Could you check a few things on this model? Use its own coordinates, in mm. Face numbers are marked on the shaded views. A direction names the side the tool comes from. Coordinates: 2 decimals unless noted, no trailing zeros. Order: outer loops, then holes, each group sorted by start corner. A loop starts at its lowest first (then second) coordinate and runs counter-clockwise, first axis right, second up. Notation, with made-up numbers: M 36,28.5 L 62,28.5 A20 ccw 62,38.5 Z; hole C 65.25,-3 d10. An arc over 180 degrees is marked long. One line per question, with ' | ' between items. Start each with the question number.
from build123d import *

# Parameters (mm, degrees)
EXTRUDE_1_DEPTH     = 11.5
FILLET_1_R          = 1
EXTRUDE_2_DEPTH     = 3.2
CUT_EXTRUDE_1_DEPTH = 1.8
CUT_EXTRUDE_2_DEPTH = 1.4


with BuildPart() as part:
    # 草图1 → 凸台-拉伸1 (new body)
    with BuildSketch(Plane(origin=(0, 0, 0), x_dir=(0, 0, -1), z_dir=(1, 0, 0))):
        Polygon((5.9, 0), (5.9, 9.85), (-5.9, 9.85), (-5.9, 0), (-7.2, 0), (-7.2, 11.15), (7.2, 11.15), (7.2, 0), align=None)
    extrude(amount=EXTRUDE_1_DEPTH)

    # 圆角1
    fillet_1_edges = [part.edges().sort_by_distance(p)[0] for p in [
        (5.75, 11.15, 7.2),
        (5.75, 11.15, -7.2),
        (5.75, 9.85, -5.9),
        (5.75, 9.85, 5.9),
    ]]
    fillet(fillet_1_edges, radius=FILLET_1_R)

    # 草图2 → 凸台-拉伸2 (add)
    with BuildSketch(Plane(origin=(0, 0, 0), x_dir=(1, 0, 0), z_dir=(0, 1, 0))):
        with BuildLine():
            Line((0, -7.2), (0, -8.8))
            ThreePointArc((0, -8.8), (4.2, -13), (8.4, -8.8))
            Line((8.4, -8.8), (8.4, -7.2))
            Line((8.4, -7.2), (0, -7.2))
        make_face()
    extrude_2 = extrude(amount=EXTRUDE_2_DEPTH)

    # 草图10 → 切除-拉伸1 (cut)
    with BuildSketch(Plane(origin=(0, 3.2, 0), x_dir=(1, 0, 0), z_dir=(0, 1, 0))):
        Polygon((7.085479679, -8.8), (6.161719249, -7.2), (2.235737418, -7.2), (1.311976987, -8.8), (2.75535266, -11.3), (5.642104006, -11.3), align=None)
    cut_extrude_1 = extrude(amount=-CUT_EXTRUDE_1_DEPTH, mode=Mode.SUBTRACT)

    # 草图11 → 切除-拉伸2 (cut)
    with BuildSketch(Plane(origin=(0, 0, 0), x_dir=(1, 0, 0), z_dir=(0, 1, 0))):
        with BuildLine():
            Line((3.087032009, -8.8), (3.087032009, -4.948738573))
            Line((3.087032009, -4.948738573), (5.337032009, -4.948738573))
            Line((5.337032009, -4.948738573), (5.337032009, -8.8))
            ThreePointArc((5.337032009, -8.8), (4.212032009, -9.925), (3.087032009, -8.8))
        make_face()
    cut_extrude_2 = extrude(amount=CUT_EXTRUDE_2_DEPTH, mode=Mode.SUBTRACT)

    # 镜向1: 凸台-拉伸2, 切除-拉伸1, 切除-拉伸2 across plane
    add(extrude_2.mirror(Plane.XY))
    add(cut_extrude_1.mirror(Plane.XY), mode=Mode.SUBTRACT)
    add(cut_extrude_2.mirror(Plane.XY), mode=Mode.SUBTRACT)


solid = part.part
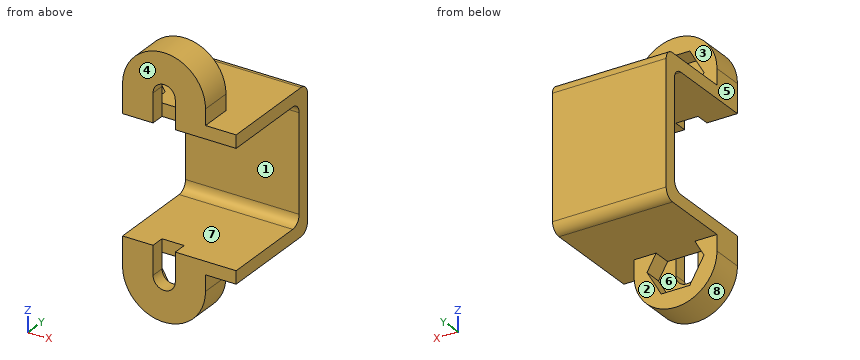
(1) Imagine slicing it at D-D, the plane z = -7.75. Write out the boundary of the cut face in (x, y), plus the area to 3 significant figures.
(2) Imagine slicing it at C-C, the plane x = 8.75. Write out the boundary of the cut face in (y, z).
(3) On a 3-axis mill with a long thin cutter (end or side, diameter ignored), from which of +Z, -Z, +X, -X, +Y, -Y can I reach the whole of each face in a straight line? I mean the marked faces 1, 2, 3 and 4. Say none if no direction works.
(4) For P1, Ø6, axis at x = 9.5, z = 3, coming from the -Y side; P2, Ø4.5, axis at x = 6, y = 6, coming from the +Z side; P3, Ø1.2, axis at x = 5, z = 8.5, coming from the +Y side; P4, Ø5, axis at x = 3.5, z = 2.5, coming from the -Y side (3 decimals), each with a flat end and sliding along its axis, tell me the tip position at first contact or that it passes through.
(5) If I drill on line 1 along Z through (x, y) = (6, 7); line 2 along Y through (x, z) = (9.25, -3.25); line 3 along X through (y, z) = (1.25, -6), over which ranges is the centre line in solid material (lowest first)? Write a range as from..to.
(6) Imagine slicing it at A-A, the plane y = 1.75. Write out the boundary of the cut face in (x, z), plus the area to 3 significant figures.
(7) We'd pull the mould along X, two halves only. Please class the marked faces 5, 6, 7 and 8: +X half, -X half, draft (parallel to the pull), parting line (faces both ways), or undercut.
(8) Imagine slicing it at B-B, the plane x = 4.2. Write out the boundary of the cut face in (y, z), plus the area to 3 significant figures.
Answers:
1) outline: M 0,0 L 3.09,0 L 3.09,1.4 L 1.92,1.4 L 1.92,3.2 L 0,3.2 Z; M 5.34,0 L 8.4,0 L 8.4,3.2 L 6.48,3.2 L 6.48,1.4 L 5.34,1.4 Z | area: 15.5 mm²
2) outline: M 0,-7.2 L 10.15,-7.2 A1 ccw 11.15,-6.2 L 11.15,6.2 A1 ccw 10.15,7.2 L 0,7.2 L 0,5.9 L 8.85,5.9 A1 cw 9.85,4.9 L 9.85,-4.9 A1 cw 8.85,-5.9 L 0,-5.9 Z
3) face 1: +X, -X, -Y | face 2: -Z, +X, -X, +Y | face 3: +Z, +X, -X, +Y | face 4: +Z, -Z, +X, -X, -Y
4) P1: y = 0 | P2: z = 7.2 | P3: y = 1.4 | P4: y = 9.845
5) line 1: -7.2..-5.9, 5.9..7.2 | line 2: 9.85..11.15 | line 3: 0..3.09, 5.34..11.5
6) outline: M 0,-8.8 A4.2 ccw 8.4,-8.8 L 8.4,-7.2 L 11.5,-7.2 L 11.5,-5.9 L 0,-5.9 Z; M 0,5.9 L 11.5,5.9 L 11.5,7.2 L 8.4,7.2 L 8.4,8.8 A4.2 ccw 0,8.8 Z; hole M 1.31,-8.8 L 2.76,-11.3 L 5.64,-11.3 L 7.09,-8.8 L 6.16,-7.2 L 2.24,-7.2 Z; hole M 1.31,8.8 L 2.24,7.2 L 6.16,7.2 L 7.09,8.8 L 5.64,11.3 L 2.76,11.3 Z | area: 75.0 mm²
7) face 5: -X half | face 6: undercut | face 7: draft | face 8: parting line
8) outline: M 0,-13 L 3.2,-13 L 3.2,-11.3 L 1.4,-11.3 L 1.4,-9.92 L 0,-9.92 Z; M 0,9.92 L 1.4,9.92 L 1.4,11.3 L 3.2,11.3 L 3.2,13 L 0,13 Z; M 1.4,-7.2 L 10.15,-7.2 A1 ccw 11.15,-6.2 L 11.15,6.2 A1 ccw 10.15,7.2 L 1.4,7.2 L 1.4,5.9 L 8.85,5.9 A1 cw 9.85,4.9 L 9.85,-4.9 A1 cw 8.85,-5.9 L 1.4,-5.9 Z | area: 55.4 mm²
